from build123d import *

# Parameters (mm, degrees)
EXTRU_MINCE1_DEPTH      = 75
ESQUISSE2_R             = 4.5
ESQUISSE2_R_2           = 1
ENL_V_MAT_EXTRU_1_DEPTH = 10
CONG_1_R                = 2
CONG_2_R                = 2
CONG_3_R                = 2
CONG_4_R                = 2
CONG_5_R                = 1
CONG_6_R                = 1
CONG_7_R                = 1
CONG_8_R                = 1
CONG_9_R                = 1
CONG_10_R               = 1
CONG_11_R               = 1
CONG_12_R               = 1


with BuildPart() as part:
    # Esquisse1 → Extru.-Mince1 (new body)
    with BuildSketch(Plane.XY):
        Polygon((-7.619194622, 27.166626694), (1.380805378, 27.166626694), (13.401620658, 15.145811413), (13.401620658, -10.854188587), (1.380805378, -22.875003867), (-7.619194622, -22.875003867), (-7.619194622, -20.875003867), (0.552378253, -20.875003867), (11.401620658, -10.025761462), (11.401620658, 14.317384289), (0.552378253, 25.166626694), (-7.619194622, 25.166626694), align=None)
    extrude(amount=EXTRU_MINCE1_DEPTH)

    # Esquisse2 → Enlèv. mat.-Extru.1 (cut)
    with BuildSketch(Plane(origin=(13.401620658, 0, 0), x_dir=(0, 0, -1), z_dir=(1, 0, 0))):
        with Locations(Location((-37.5, 2.145811413, 0), (0, 0, 90))):
            Circle(ESQUISSE2_R)
        with Locations(Location((-46.5, 2.145811413, 0), (0, 0, 90))):
            Circle(ESQUISSE2_R_2)
        with Locations(Location((-28.5, 2.145811413, 0), (0, 0, 90))):
            Circle(ESQUISSE2_R_2)
        with Locations(Location((-37.5, 11.145811413, 0), (0, 0, 90))):
            Circle(ESQUISSE2_R_2)
        with Locations(Location((-37.5, -6.854188587, 0), (0, 0, 90))):
            Circle(ESQUISSE2_R_2)
    extrude(amount=-ENL_V_MAT_EXTRU_1_DEPTH, mode=Mode.SUBTRACT)

    # Congé1
    cong_1_edges = [part.edges().sort_by_distance(p)[0] for p in [
        (-7.619194622, 26.166626694, 0),
    ]]
    fillet(cong_1_edges, radius=CONG_1_R)

    # Congé2
    cong_2_edges = [part.edges().sort_by_distance(p)[0] for p in [
        (-7.619194622, -21.875003867, 0),
    ]]
    fillet(cong_2_edges, radius=CONG_2_R)

    # Congé3
    cong_3_edges = [part.edges().sort_by_distance(p)[0] for p in [
        (-7.619194622, -21.875003867, 75),
    ]]
    fillet(cong_3_edges, radius=CONG_3_R)

    # Congé4
    cong_4_edges = [part.edges().sort_by_distance(p)[0] for p in [
        (-7.619194622, 26.166626694, 75),
    ]]
    fillet(cong_4_edges, radius=CONG_4_R)

    # Congé5
    cong_5_edges = [part.edges().sort_by_distance(p)[0] for p in [
        (11.401620658, 14.317384289, 37.5),
    ]]
    fillet(cong_5_edges, radius=CONG_5_R)

    # Congé6
    cong_6_edges = [part.edges().sort_by_distance(p)[0] for p in [
        (11.401620658, -10.025761462, 37.5),
    ]]
    fillet(cong_6_edges, radius=CONG_6_R)

    # Congé7
    cong_7_edges = [part.edges().sort_by_distance(p)[0] for p in [
        (13.401620658, -10.854188587, 37.5),
    ]]
    fillet(cong_7_edges, radius=CONG_7_R)

    # Congé8
    cong_8_edges = [part.edges().sort_by_distance(p)[0] for p in [
        (13.401620658, 15.145811413, 37.5),
    ]]
    fillet(cong_8_edges, radius=CONG_8_R)

    # Congé9
    cong_9_edges = [part.edges().sort_by_distance(p)[0] for p in [
        (1.380805378, 27.166626694, 37.5),
    ]]
    fillet(cong_9_edges, radius=CONG_9_R)

    # Congé10
    cong_10_edges = [part.edges().sort_by_distance(p)[0] for p in [
        (1.380805378, -22.875003867, 37.5),
    ]]
    fillet(cong_10_edges, radius=CONG_10_R)

    # Congé11
    cong_11_edges = [part.edges().sort_by_distance(p)[0] for p in [
        (0.552378253, 25.166626694, 37.5),
    ]]
    fillet(cong_11_edges, radius=CONG_11_R)

    # Congé12
    cong_12_edges = [part.edges().sort_by_distance(p)[0] for p in [
        (0.552378253, -20.875003867, 37.5),
    ]]
    fillet(cong_12_edges, radius=CONG_12_R)


solid = part.part
Verification items for the finished model (mm, model axes). A direction names the side the tool comes from. Round coordinates to 2 decimals unless told otherwise and drop trailing zeros. Order: outer loops, then holes, each group sorted by start corner. A loop starts at its lowest first (then second) coordinate and runs counter-clockwise, first axis right, second up.
1. Access from +Z, -Z, +X, -X, +Y, -Y to the whole of each face (thin tool, end or side, straight path). Record for faces 5 (the flat face through (-4, -20.875, 37)), 6 (the flat face through (-7.619, -22, 37)).
Final values:
face 5: +Z, -Z, -X
face 6: +Z, -Z, -X, +Y, -Y
2. Section check C-C on x = -3.75. Record the cut outline in (y, z) (3 decimals), then the cut area to 3 significant figures.
Final values:
outline: (-22.875, 0) - (-20.875, 0) - (-20.875, 75) - (-22.875, 75) - close; (25.167, 0) - (27.167, 0) - (27.167, 75) - (25.167, 75) - close
area: 300 mm2
3. Release check for a two-part mould opening along Y. For faces 1 (the flat face through (-3, 27.167, 37)), 2 (the flat face through (6.05, 19.67, 36.98)), 3 (the cylindrical face through (12.416, 11.683, 38.343)), 4 (the flat face through (-3, -22.875, 37)) record: +Y half, -Y half, draft (parallel to the pull), parting line (faces both ways), or undercut.
Final values:
face 1: +Y half
face 2: undercut
face 3: undercut
face 4: -Y half
4. Go/stop test with flat-tipped pins: P1, Ø12, axis at y = -10, z = 56.5, coming from the -X side; P2, Ø5, axis at y = -2.5, z = 65.5, coming from the -X side; P3, Ø10, axis at y = 21.5, z = 11, coming from the +X side. Record where each tip stops, or that it passes through.
Final values:
P1: stops at x = 5.43
P2: stops at x = 11.4
P3: stops at x = 12.05
5. Section check D-D on y = -7. Record the cut outline in (x, z).
Final values:
outline: (11.4, 0) - (13.4, 0) - (13.4, 36.51) - (11.4, 36.51) - close; (11.4, 38.49) - (13.4, 38.49) - (13.4, 75) - (11.4, 75) - close
6. Section check A-A on z = 37.5. State how many separate pieces and enclosed holes the cut face has, then the cut area to 3 significant figures.
Final values:
separate pieces: 4
enclosed holes: 0
area: 123 mm2
7. Thickness scan on L1, parallel to Y at x = -5.25, z = 22.5 (3 decimals); L2, parallel to X at y = 4.5, z = 59; L3, parallel to Y at x = 1.5, z = 32. Record the ranges inside material, lowest first.
Final values:
L1: y = -22.875 to -20.875, 25.167 to 27.167
L2: x = 11.4 to 13.4
L3: y = -22.72 to -19.93, 24.22 to 27.01
8. Section check B-B on z = 46.5. Record the cut outline in (x, y) (3 decimals).
Final values:
outline: (-7.619, -22.875) - (0.967, -22.875) arc R1 ccw to (1.674, -22.582) - (13.109, -11.147) arc R1 ccw to (13.402, -10.44) - (13.402, 1.146) - (11.402, 1.146) - (11.402, -9.612) arc R1 cw to (11.109, -10.319) - (0.845, -20.582) arc R1 cw to (0.138, -20.875) - (-7.619, -20.875) - close; (-7.619, 25.167) - (0.138, 25.167) arc R1 cw to (0.845, 24.874) - (11.109, 14.61) arc R1 cw to (11.402, 13.903) - (11.402, 3.146) - (13.402, 3.146) - (13.402, 14.732) arc R1 ccw to (13.109, 15.439) - (1.674, 26.874) arc R1 ccw to (0.967, 27.167) - (-7.619, 27.167) - close
